For this review, take the finished solid that the model builds, in its own axes (mm). A direction names the side the tool comes from. Round coordinates to 2 decimals unless told otherwise and drop trailing zeros. Order: outer loops, then holes, each group sorted by start corner. A loop starts at its lowest first (then second) coordinate and runs counter-clockwise, first axis right, second up. Notation, with made-up numbers: M 28,83.5 L 41,83.5 A18 ccw 41,101.5 Z; hole C 60,64 d4. An arc over 180 degrees is marked long. Use a Markdown table: item, result.
from build123d import *

# Parameters (mm, degrees)
SKETCH1_R           = 1.65
BOSS_EXTRUDE1_DEPTH = 3.5


with BuildPart() as part:
    # Sketch1 → Boss-Extrude1 (new body)
    with BuildSketch(Plane(origin=(0, 0, 0), x_dir=(1, 0, 0), z_dir=(0, 1, 0))):
        with BuildLine():
            ThreePointArc((-75, 38), (-74.414213562, 39.414213562), (-73, 40))
            Line((-73, 40), (73, 40))
            ThreePointArc((73, 40), (74.414213562, 39.414213562), (75, 38))
            Line((75, 38), (75, -38))
            ThreePointArc((75, -38), (74.414213562, -39.414213562), (73, -40))
            Line((73, -40), (-73, -40))
            ThreePointArc((-73, -40), (-74.414213562, -39.414213562), (-75, -38))
            Line((-75, -38), (-75, 38))
        make_face()
        with Locations(Location((71.542893219, 36.542893219, 0), (0, 0, 270))):
            Circle(SKETCH1_R, mode=Mode.SUBTRACT)
        with Locations(Location((-71.542893219, 36.542893219, 0), (0, 0, 270))):
            Circle(SKETCH1_R, mode=Mode.SUBTRACT)
        with Locations(Location((71.542893219, -36.552437932, 0), (0, 0, 270))):
            Circle(SKETCH1_R, mode=Mode.SUBTRACT)
        with Locations(Location((-71.542893219, -36.552437932, 0), (0, 0, 270))):
            Circle(SKETCH1_R, mode=Mode.SUBTRACT)
        with BuildLine():
            ThreePointArc((-46, 27.948088576), (-50, 31.948088576), (-54, 27.948088576))
            Line((-54, 27.948088576), (-54, -27.957633289))
            ThreePointArc((-54, -27.957633289), (-50, -31.957633289), (-46, -27.957633289))
            Line((-46, -27.957633289), (-46, 27.948088576))
        make_face(mode=Mode.SUBTRACT)
        with BuildLine():
            ThreePointArc((-21, 27.948088576), (-25, 31.948088576), (-29, 27.948088576))
            Line((-29, 27.948088576), (-29, -27.957633289))
            ThreePointArc((-29, -27.957633289), (-25, -31.957633289), (-21, -27.957633289))
            Line((-21, -27.957633289), (-21, 27.948088576))
        make_face(mode=Mode.SUBTRACT)
        with BuildLine():
            ThreePointArc((54, 27.948088576), (50, 31.948088576), (46, 27.948088576))
            Line((46, 27.948088576), (46, -27.957633289))
            ThreePointArc((46, -27.957633289), (50, -31.957633289), (54, -27.957633289))
            Line((54, -27.957633289), (54, 27.948088576))
        make_face(mode=Mode.SUBTRACT)
        with BuildLine():
            ThreePointArc((29, 27.948088576), (25, 31.948088576), (21, 27.948088576))
            Line((21, 27.948088576), (21, -27.957633289))
            ThreePointArc((21, -27.957633289), (25, -31.957633289), (29, -27.957633289))
            Line((29, -27.957633289), (29, 27.948088576))
        make_face(mode=Mode.SUBTRACT)
        with BuildLine():
            ThreePointArc((4, 27.948088576), (0, 31.948088576), (-4, 27.948088576))
            Line((-4, 27.948088576), (-4, -27.957633289))
            ThreePointArc((-4, -27.957633289), (0, -31.957633289), (4, -27.957633289))
            Line((4, -27.957633289), (4, 27.948088576))
        make_face(mode=Mode.SUBTRACT)
    extrude(amount=BOSS_EXTRUDE1_DEPTH)


solid = part.part
Q1. Add section A-A (x = 0). Write out the cut boundary in (y, z).
Determined:
| item | result |
|---|---|
| outline | M 0,-40 L 3.5,-40 L 3.5,-31.95 L 0,-31.95 Z; M 0,31.96 L 3.5,31.96 L 3.5,40 L 0,40 Z |
Q2. Add section B-B (z = 19.5). Write out the cut boundary in (x, y), then the cut area to 3 significant figures.
Determined:
| item | result |
|---|---|
| outline | M -75,0 L -54,0 L -54,3.5 L -75,3.5 Z; M -46,0 L -29,0 L -29,3.5 L -46,3.5 Z; M -21,0 L -4,0 L -4,3.5 L -21,3.5 Z; M 4,0 L 21,0 L 21,3.5 L 4,3.5 Z; M 29,0 L 46,0 L 46,3.5 L 29,3.5 Z; M 54,0 L 75,0 L 75,3.5 L 54,3.5 Z |
| area | 385 mm^2 |
Q3. Draft analysis for pull direction Z (two halves, no side actions). For faces 3 (the flat face through (21, 2, 0)), 4 (the flat face through (-1, 2, -40)), 5 (the flat face through (18, 3.5, -1)), state which applies: pulls with the +Z half, pulls with the -Z half, needs draft (parallel to the pull), parting line crosses it, or undercut.
Determined:
| item | result |
|---|---|
| face 3 | undercut |
| face 4 | pulls with the -Z half |
| face 5 | needs draft |
Q4. Machinability: for faces 1 (the flat face through (46, 2, 0)), 2 (the flat face through (18, 0, -1)), which of the approach directions +Z, -Z, +X, -X, +Y, -Y give a long, thin tool a straight path to every point of the face, cutting with its end or side? Answer none if there is none.
Determined:
| item | result |
|---|---|
| face 1 | +Y, -Y |
| face 2 | +Z, -Z, +X, -X, -Y |
Q5. Clearance check with flat-ended pins moving along their axes: pin 1 (3 mm diameter, centred on x = 71.54, z = 36.55, fed in from +Y); pin 2 (4.5 mm diameter, centred on x = -71.54, z = -36.54, fed in from -Y). State where each tip first meets the part, or that it passes through.
Determined:
| item | result |
|---|---|
| pin 1 | passes through |
| pin 2 | stops at y = 0 |
Q6. Wall thickness on line 1 along X through (y, z) = (1.35, -26); line 2 along X through (y, z) = (3.2, 30); line 3 along X through (y, z) = (0.2, 36.5): over which ranges is each line inside the solid? List them lowest first. Write a range as [from, to].
Determined:
| item | result |
|---|---|
| line 1 | x = [-75, -54], [-46, -29], [-21, -4], [4, 21], [29, 46], [54, 75] |
| line 2 | x = [-75, -53.44], [-46.56, -28.44], [-21.56, -3.44], [3.44, 21.56], [28.44, 46.56], [53.44, 75] |
| line 3 | x = [-75, -73.19], [-69.89, 69.89], [73.19, 75] |
Q7. Add section C-C (y = 1.1). Give the number of separate pieces and of enclosed holes in the cut face, then the cut area to 3 significant figures.
Determined:
| item | result |
|---|---|
| separate pieces | 1 |
| enclosed holes | 9 |
| area | 9,470 mm^2 |
Q8. Add section D-D (x = 27.5). Write out the cut boundary in (y, z).
Determined:
| item | result |
|---|---|
| outline | M 0,-40 L 3.5,-40 L 3.5,-31.07 L 0,-31.07 Z; M 0,31.08 L 3.5,31.08 L 3.5,40 L 0,40 Z |
